Check sheet for the modelled part. Datum: model origin and axes. Units: mm. Face numbers are marked on the shaded views. A direction names the side the tool comes from. Coordinates: 2 decimals unless noted, no trailing zeros. Loops run counter-clockwise (first coordinate to the right, second up) from the corner with the lowest first, then second, coordinate; pieces in that order, holes last.
from build123d import *

# Parameters (mm, degrees)
SKETCH1_R                  = 4.5
EXTRUDE1_DEPTH             = 2
PROCESS_BENDS1_START       = -58
PROCESS_BENDS1_OUTLINE_W   = 25
PROCESS_BENDS1_OUTLINE_H   = 2
PROCESS_BENDS1_DEPTH       = 40.887009382
PROCESS_BENDS1_START_2     = 17.112990618
PROCESS_BENDS1_2_OUTLINE_W = 25
PROCESS_BENDS1_2_OUTLINE_H = 2
PROCESS_BENDS1_2_DEPTH     = 40.887009382
PROCESS_BENDS1_START_3     = 13.596613306
PROCESS_BENDS1_3_OUTLINE_R = 4.5
PROCESS_BENDS1_3_DEPTH     = 9.345511755
PROCESS_BENDS1_START_4     = -22.942125061
PROCESS_BENDS1_4_OUTLINE_R = 4.5
PROCESS_BENDS1_4_DEPTH     = 9.157953378
PROCESS_BENDS1_START_5     = -12.5
PROCESS_BENDS1_5_DEPTH     = 25
PROCESS_BENDS1_6_DEPTH     = 25


with BuildPart() as part:
    # Sketch1 → Extrude1 (new body)
    with BuildSketch(Plane.XY):
        with BuildLine():
            Line((-45, 12.5), (45, 12.5))
            ThreePointArc((45, 12.5), (57.5, 0), (45, -12.5))
            Line((45, -12.5), (-45, -12.5))
            ThreePointArc((-45, -12.5), (-57.5, 0), (-45, 12.5))
        make_face()
        with Locations((45, 0)):
            Circle(SKETCH1_R, mode=Mode.SUBTRACT)
        with Locations(Location((-45, 0, 0), (0, 0, 180))):
            Circle(SKETCH1_R, mode=Mode.SUBTRACT)
        Circle(SKETCH1_R, mode=Mode.SUBTRACT)
    extrude(amount=EXTRUDE1_DEPTH)

    # Process-Bends1: read off the stored shape, not the designer's step
    # Process-Bends1 outline → Process-Bends1 (cut)
    with BuildSketch(Plane.YZ.offset(PROCESS_BENDS1_START)):
        with Locations((0, 1)):
            Rectangle(PROCESS_BENDS1_OUTLINE_W, PROCESS_BENDS1_OUTLINE_H)
    extrude(amount=PROCESS_BENDS1_DEPTH, mode=Mode.SUBTRACT)

    # Process-Bends1 2 outline → Process-Bends1 2 (cut)
    with BuildSketch(Plane.YZ.offset(PROCESS_BENDS1_START_2)):
        with Locations((0, 1)):
            Rectangle(PROCESS_BENDS1_2_OUTLINE_W, PROCESS_BENDS1_2_OUTLINE_H)
    extrude(amount=PROCESS_BENDS1_2_DEPTH, mode=Mode.SUBTRACT)

    # Process-Bends1 3 outline → Process-Bends1 3 (add)
    with BuildSketch(Plane.YZ.offset(PROCESS_BENDS1_START_3)):
        with BuildLine():
            ThreePointArc((12.5, 30.115293784), (0, 42.615293784), (-12.5, 30.115293784))
            Line((-12.5, 30.115293784), (-12.5, 2))
            Line((-12.5, 2), (12.5, 2))
            Line((12.5, 2), (12.5, 30.115293784))
        make_face()
        with Locations((0, 30.115293784)):
            Circle(PROCESS_BENDS1_3_OUTLINE_R, mode=Mode.SUBTRACT)
    extrude(amount=PROCESS_BENDS1_3_DEPTH)

    # Process-Bends1 4 outline → Process-Bends1 4 (add)
    with BuildSketch(Plane.YZ.offset(PROCESS_BENDS1_START_4)):
        with BuildLine():
            ThreePointArc((12.5, 30.115293784), (0, 42.615293784), (-12.5, 30.115293784))
            Line((-12.5, 30.115293784), (-12.5, 2))
            Line((-12.5, 2), (12.5, 2))
            Line((12.5, 2), (12.5, 30.115293784))
        make_face()
        with Locations((0, 30.115293784)):
            Circle(PROCESS_BENDS1_4_OUTLINE_R, mode=Mode.SUBTRACT)
    extrude(amount=PROCESS_BENDS1_4_DEPTH)

    # Process-Bends1 5 outline → Process-Bends1 5 (cut)
    with BuildSketch(Plane(origin=(0, 0, 0), x_dir=(1, 0, 0), z_dir=(0, 1, 0)).offset(PROCESS_BENDS1_START_5)):
        with BuildLine():
            ThreePointArc((-20.754740635, -14.851688233), (-20.894717075, -15.264045529), (-20.942125061, -15.696924757))
            Line((-20.942125061, -15.696924757), (-20.942125061, -44))
            Line((-20.942125061, -44), (-13.784171683, -44))
            Line((-13.784171683, -44), (-13.784171683, -2.022087009))
            ThreePointArc((-13.784171683, -2.022087009), (-14.684730041, -2.397732403), (-15.300375044, -3.154763477))
            Line((-15.300375044, -3.154763477), (-20.754740635, -14.851688233))
        make_face()
        with BuildLine():
            Line((13.596613306, -2.002964486), (13.596613306, -44))
            Line((13.596613306, -44), (20.942125061, -44))
            Line((20.942125061, -44), (20.942125061, -15.696924757))
            ThreePointArc((20.942125061, -15.696924757), (20.894717075, -15.264045529), (20.754740635, -14.851688233))
            Line((20.754740635, -14.851688233), (15.300375044, -3.154763477))
            ThreePointArc((15.300375044, -3.154763477), (14.607880625, -2.343096684), (13.596613306, -2.002964486))
        make_face()
        with BuildLine():
            Line((-22.942125061, -2), (-22.942125061, -15.696924757))
            ThreePointArc((-22.942125061, -15.696924757), (-22.847309089, -14.831166301), (-22.567356209, -14.00645171))
            Line((-22.567356209, -14.00645171), (-17.112990618, -2.309526953))
            ThreePointArc((-17.112990618, -2.309526953), (-15.636957903, -0.626434217), (-13.48775947, 0))
            Line((-13.48775947, 0), (-17.112990618, 0))
            Line((-17.112990618, 0), (-17.112990618, -2))
            Line((-17.112990618, -2), (-22.942125061, -2))
        make_face()
        with BuildLine():
            Line((22.942125061, -2), (17.112990618, -2))
            Line((17.112990618, -2), (17.112990618, 0))
            Line((17.112990618, 0), (13.48775947, 0))
            ThreePointArc((13.48775947, 0), (15.636957903, -0.626434217), (17.112990618, -2.309526953))
            Line((17.112990618, -2.309526953), (22.567356209, -14.00645171))
            ThreePointArc((22.567356209, -14.00645171), (22.847309089, -14.831166301), (22.942125061, -15.696924757))
            Line((22.942125061, -15.696924757), (22.942125061, -2))
        make_face()
    extrude(amount=PROCESS_BENDS1_5_DEPTH, mode=Mode.SUBTRACT)

    # Process-Bends1 6 outline → Process-Bends1 6 (add)
    with BuildSketch(Plane(origin=(0, 0, 0), x_dir=(1, 0, 0), z_dir=(0, 1, 0)).offset(PROCESS_BENDS1_START_5)):
        with BuildLine():
            Line((-13.784171683, -2), (-13.784171683, -2.022087009))
            ThreePointArc((-13.784171683, -2.022087009), (-13.636376458, -2.005529396), (-13.48775947, -2))
            Line((-13.48775947, -2), (-13.784171683, -2))
        make_face()
        with BuildLine():
            Line((13.596613306, -2.000000001), (13.48775947, -2))
            ThreePointArc((13.48775947, -2), (13.542206568, -2.000741259), (13.596613306, -2.002964486))
            Line((13.596613306, -2.002964486), (13.596613306, -2.000000001))
        make_face()
    extrude(amount=PROCESS_BENDS1_6_DEPTH)


solid = part.part
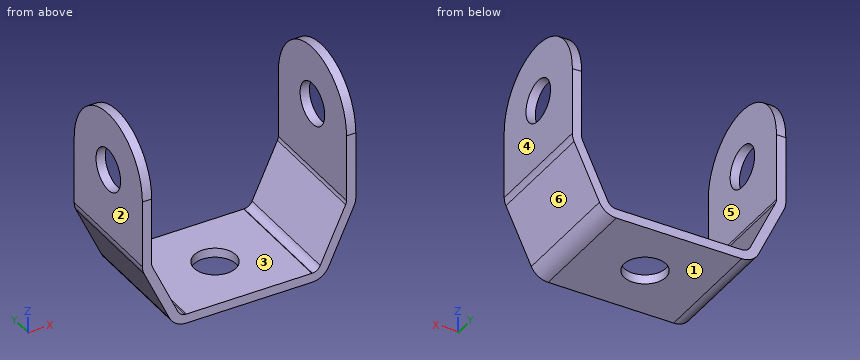
(1) Section check B-B, the plane y = 2.25. Count the separate pieces of the cut face and the enclosed holes in it, plus the area to 3 significant figures.
(2) Scan lines: line 1 along X through (y, z) = (-7, 38.5); line 2 along Y through (x, z) = (0, 1.5); line 3 along Z through (x, y) = (7, 1.5). Record each from-to range of solid material in increasing order.
(3) Section check D-D, the plane y = 8.25. Enter the section's corners in (x, z), plus the area to 3 significant figures.
(4) Section check A-A, the plane x = 0. Enter the section's corners in (y, z), plus the area to 3 significant figures.
(5) Gauge pin test, flat ends, axial feed: P1, Ø10, axis at x = -9, y = -8.5, coming from the +Z side; P2, Ø8, axis at y = 7.5, z = 5.5, coming from the -X side; P3, Ø7.5, axis at x = 2, y = 2, coming from the +Z side. Record the tip position at first contact, or that the pin passes through.
(6) Section check C-C, the plane z = 37.5. Enter the section's corners in (x, y).
(7) Set-up check for the marked faces 5 and 6: record each of +Z, -Z, +X, -X, +Y, -Y from which the full face is reachable in a straight line by a thin tool's end or side.
(8) Draft check along X on the marked faces 1, 2, 3 and 4. Enter one of: pulls with the +X half, pulls with the -X half, needs draft (parallel to the pull), parting line crosses it, or undercut.
Determined:
1. separate pieces: 4
1. enclosed holes: 0
1. area: 185 mm2
2. line 1: x = -22.94 to -20.94, 20.94 to 22.94
2. line 2: y = -12.5 to -4.5, 4.5 to 12.5
2. line 3: z = 0 to 2
3. outline: (-22.94, 15.7) arc R4 ccw to (-22.57, 14.01) - (-17.11, 2.31) arc R4 ccw to (-13.49, 0) - (13.49, 0) arc R4 ccw to (17.11, 2.31) - (22.57, 14.01) arc R4 ccw to (22.94, 15.7) - (22.94, 39.51) - (20.94, 39.51) - (20.94, 15.7) arc R2 cw to (20.75, 14.85) - (15.3, 3.15) arc R2 cw to (13.49, 2) - (-13.49, 2) arc R2 cw to (-15.3, 3.15) - (-20.75, 14.85) arc R2 cw to (-20.94, 15.7) - (-20.94, 39.51) - (-22.94, 39.51) - close
3. area: 220 mm2
4. outline: (-12.5, 0) - (-4.5, 0) - (-4.5, 2) - (-12.5, 2) - close; (4.5, 0) - (12.5, 0) - (12.5, 2) - (4.5, 2) - close
4. area: 32.0 mm2
5. P1: stops at z = 2.07
5. P2: stops at x = -20.47
5. P3: stops at z = 2
6. outline: (-22.94, -10.09) - (-20.94, -10.09) - (-20.94, 10.09) - (-22.94, 10.09) - close; (20.94, -10.09) - (22.94, -10.09) - (22.94, 10.09) - (20.94, 10.09) - close
7. face 5: +Z, +Y, -Y
7. face 6: -Z, +X, +Y, -Y
8. face 1: needs draft
8. face 2: pulls with the -X half
8. face 3: undercut
8. face 4: pulls with the +X half
